from build123d import *

# Parameters (mm, degrees)
PROFILE_DEPTH       = 50
SLOT_DEPTH          = 54.434539392
SLOTLP_COUNT        = 3
SLOTLP_PITCH        = 20
SLOTHP_COPY_1_DEPTH = 54.434539392
SLOTHP_COPY_2_DEPTH = 54.434539392
SLOTHP_COPY_3_DEPTH = 54.434539392


with BuildPart() as part:
    # ProfileS → Profile (new, symmetric)
    with BuildSketch(Plane(origin=(0, 0, 0), x_dir=(0, 0, -1), z_dir=(1, 0, 0))):
        with BuildLine():
            Line((-13.5, 0), (13.5, 0))
            ThreePointArc((13.5, 0), (13.853553391, 0.146446609), (14, 0.5))
            Line((14, 0.5), (14, 5.9))
            ThreePointArc((14, 5.9), (14.029289322, 5.970710678), (14.1, 6))
            Line((14.1, 6), (17.3, 6))
            ThreePointArc((17.3, 6), (17.441421356, 6.058578644), (17.5, 6.2))
            Line((17.5, 6.2), (17.5, 6.8))
            ThreePointArc((17.5, 6.8), (17.441421356, 6.941421356), (17.3, 7))
            Line((17.3, 7), (13.1, 7))
            ThreePointArc((13.1, 7), (13.029289322, 6.970710678), (13, 6.9))
            Line((13, 6.9), (13, 1.1))
            ThreePointArc((13, 1.1), (12.970710678, 1.029289322), (12.9, 1))
            Line((12.9, 1), (-12.9, 1))
            ThreePointArc((-12.9, 1), (-12.970710678, 1.029289322), (-13, 1.1))
            Line((-13, 1.1), (-13, 6.9))
            ThreePointArc((-13, 6.9), (-13.029289322, 6.970710678), (-13.1, 7))
            Line((-13.1, 7), (-17.3, 7))
            ThreePointArc((-17.3, 7), (-17.441421356, 6.941421356), (-17.5, 6.8))
            Line((-17.5, 6.8), (-17.5, 6.2))
            ThreePointArc((-17.5, 6.2), (-17.441421356, 6.058578644), (-17.3, 6))
            Line((-17.3, 6), (-14.1, 6))
            ThreePointArc((-14.1, 6), (-14.029289322, 5.970710678), (-14, 5.9))
            Line((-14, 5.9), (-14, 0.5))
            ThreePointArc((-14, 0.5), (-13.853553391, 0.146446609), (-13.5, 0))
        make_face()
    extrude(amount=PROFILE_DEPTH, both=True)

    # SlotS → Slot (cut, through all)
    with BuildSketch(Plane(origin=(0, 0, 0), x_dir=(1, 0, 0), z_dir=(0, 1, 0))):
        with BuildLine():
            Line((-3.95, 2.05), (3.95, 2.05))
            ThreePointArc((3.95, 2.05), (6, 0), (3.95, -2.05))
            Line((3.95, -2.05), (-3.95, -2.05))
            ThreePointArc((-3.95, -2.05), (-6, 0), (-3.95, 2.05))
        make_face()
    slot = extrude(amount=SLOT_DEPTH, mode=Mode.SUBTRACT)

    # SlotLP: Slot ×3
    with Locations(*[(-i * SLOTLP_PITCH, 0, 0) for i in range(1, SLOTLP_COUNT)]):
        add(slot, mode=Mode.SUBTRACT)

    # SlotHP copy 1 sketch → SlotHP copy 1 (cut, through all)
    with BuildSketch(Plane(origin=(20, 0, 0), x_dir=(-1, 0, 0), z_dir=(0, 1, 0))):
        with BuildLine():
            Line((-3.95, -2.05), (3.95, -2.05))
            ThreePointArc((3.95, -2.05), (6, 0), (3.95, 2.05))
            Line((3.95, 2.05), (-3.95, 2.05))
            ThreePointArc((-3.95, 2.05), (-6, 0), (-3.95, -2.05))
        make_face()
    extrude(amount=SLOTHP_COPY_1_DEPTH, mode=Mode.SUBTRACT)

    # SlotHP copy 2 sketch → SlotHP copy 2 (cut, through all)
    with BuildSketch(Plane(origin=(40, 0, 0), x_dir=(-1, 0, 0), z_dir=(0, 1, 0))):
        with BuildLine():
            Line((-3.95, -2.05), (3.95, -2.05))
            ThreePointArc((3.95, -2.05), (6, 0), (3.95, 2.05))
            Line((3.95, 2.05), (-3.95, 2.05))
            ThreePointArc((-3.95, 2.05), (-6, 0), (-3.95, -2.05))
        make_face()
    extrude(amount=SLOTHP_COPY_2_DEPTH, mode=Mode.SUBTRACT)

    # SlotHP copy 3 sketch → SlotHP copy 3 (cut, through all)
    with BuildSketch(Plane(origin=(0, 0, 0), x_dir=(-1, 0, 0), z_dir=(0, 1, 0))):
        with BuildLine():
            Line((-3.95, -2.05), (3.95, -2.05))
            ThreePointArc((3.95, -2.05), (6, 0), (3.95, 2.05))
            Line((3.95, 2.05), (-3.95, 2.05))
            ThreePointArc((-3.95, 2.05), (-6, 0), (-3.95, -2.05))
        make_face()
    extrude(amount=SLOTHP_COPY_3_DEPTH, mode=Mode.SUBTRACT)


solid = part.part
Build history of the part. All positions in model axes, mm. A direction names the side the tool comes from. Give positions to 0.01 mm unless a question says otherwise; leave off trailing zeros. Write each loop counter-clockwise with the first axis right and the second up, starting at its lowest first coordinate (ties: lowest second). Pieces come first, ordered by that corner, then holes. Notation, with made-up numbers: (19, 74) - (33, 74) arc R15 ccw to (33, 81) - close; hole circle Ø1 at (37.5, -15). An arc over 180 degrees is marked (long way). Use one line per item in the form item = value. Start each with the question number.
1. 3-axis set-ups, long thin cutter, end or side, ignore diameter. For faces 1 (the face through (14, 0.5, 0)), 2 (the face through (1, 3, -14)), 3 (the face through (1, 4, -13)), 4 (the face through (1, 3, 14)): which of +Z, -Z, +X, -X, +Y, -Y reach the whole face in a straight line?
2. Drop flat-ended pins along their axis: pin 1 Ø1.1 at (x, y) = (-21, 0.5) entering from +Z; pin 2 Ø1.1 at (x, y) = (20, 0.5) entering from -Z; pin 3 Ø1 at (x, z) = (9.5, -16.5) entering from -Y; pin 4 Ø4 at (y, z) = (5.5, -9.5) entering from -X. Give the stop position or say it passes through.
3. Band-saw the part on B-B on y = 3. Write the cut outline in (x, z).
4. Probe line 1 (Z direction, x = -30.5, y = 3.5); line 2 (Z direction, x = -7.5, y = 6.75); line 3 (Z direction, x = -12.5, y = 0.75). List the from-to ranges inside material, lowest first. Write a range as [from, to].
5. Band-saw the part on D-D on z = 3.5. Write the cut outline in (x, y), plus the area to 3 significant figures.
6. Band-saw the part on C-C on x = 12.5. Write the cut outline in (y, z), plus the area to 3 significant figures.
7. Band-saw the part on A-A on x = -1. Write the cut outline in (y, z).
8. Two-plate mould, pull along X, no slides. Class faces 5 (the face through (-26, 0.5, 0)), 6 (the face through (1, 0, 3)), 7 (the face through (-50, 0.4, 2.7)): released by +X, released by -X, zero draft, split by the parting line, or undercut.
Conclusion:
q1.face_1 = +Y, -Y
q1.face_2 = -Z, +X, -X, -Y
q1.face_3 = +X, -X, +Y
q1.face_4 = +Z, +X, -X, -Y
q2.pin_1 = 14
q2.pin_2 = -14
q2.pin_3 = 6
q2.pin_4 = through
q3.outline = (-50, -14) - (50, -14) - (50, -13) - (-50, -13) - close; (-50, 13) - (50, 13) - (50, 14) - (-50, 14) - close
q4.line_1 = [-14, -13], [13, 14]
q4.line_2 = [-17.5, -13], [13, 17.5]
q4.line_3 = [-14, 14]
q5.outline = (-50, 0) - (50, 0) - (50, 1) - (-50, 1) - close
q5.area = 100 mm²
q6.outline = (0, -13.5) arc R0.5 ccw to (0.5, -14) - (5.9, -14) arc R0.1 cw to (6, -14.1) - (6, -17.3) arc R0.2 ccw to (6.2, -17.5) - (6.8, -17.5) arc R0.2 ccw to (7, -17.3) - (7, -13.1) arc R0.1 ccw to (6.9, -13) - (1.1, -13) arc R0.1 cw to (1, -12.9) - (1, 12.9) arc R0.1 cw to (1.1, 13) - (6.9, 13) arc R0.1 ccw to (7, 13.1) - (7, 17.3) arc R0.2 ccw to (6.8, 17.5) - (6.2, 17.5) arc R0.2 ccw to (6, 17.3) - (6, 14.1) arc R0.1 cw to (5.9, 14) - (0.5, 14) arc R0.5 ccw to (0, 13.5) - close
q6.area = 46.9 mm²
q7.outline = (0, -13.5) arc R0.5 ccw to (0.5, -14) - (5.9, -14) arc R0.1 cw to (6, -14.1) - (6, -17.3) arc R0.2 ccw to (6.2, -17.5) - (6.8, -17.5) arc R0.2 ccw to (7, -17.3) - (7, -13.1) arc R0.1 ccw to (6.9, -13) - (1.1, -13) arc R0.1 cw to (1, -12.9) - (1, -2.05) - (0, -2.05) - close; (0, 2.05) - (1, 2.05) - (1, 12.9) arc R0.1 cw to (1.1, 13) - (6.9, 13) arc R0.1 ccw to (7, 13.1) - (7, 17.3) arc R0.2 ccw to (6.8, 17.5) - (6.2, 17.5) arc R0.2 ccw to (6, 17.3) - (6, 14.1) arc R0.1 cw to (5.9, 14) - (0.5, 14) arc R0.5 ccw to (0, 13.5) - close
q8.face_5 = undercut
q8.face_6 = zero draft
q8.face_7 = released by -X
